Design review of the part built by this model. Coordinates are the model's own, in mm. A direction names the side the tool comes from. Round coordinates to 2 decimals unless told otherwise and drop trailing zeros. Write each loop counter-clockwise with the first axis right and the second up, starting at its lowest first coordinate (ties: lowest second). Pieces come first, ordered by that corner, then holes.
from build123d import *

# Parameters (mm, degrees)
SKETCH1_W           = 400
SKETCH1_H           = 300
BOSS_EXTRUDE1_DEPTH = 10
SKETCH2_W           = 8
SKETCH2_H           = 30
BOSS_EXTRUDE2_DEPTH = 40
SKETCH3_R           = 5
CUT_EXTRUDE1_DEPTH  = 374.607079697
FILLET1_R           = 15
SKETCH4_W           = 8
SKETCH4_H           = 30
BOSS_EXTRUDE3_DEPTH = 40
SKETCH5_R           = 5
CUT_EXTRUDE2_DEPTH  = 374.607079697
FILLET2_R           = 15


with BuildPart() as part:
    # Sketch1 → Boss-Extrude1 (new body)
    with BuildSketch(Plane(origin=(0, 0, 0), x_dir=(1, 0, 0), z_dir=(0, 1, 0))):
        Rectangle(SKETCH1_W, SKETCH1_H)
    extrude(amount=BOSS_EXTRUDE1_DEPTH)

    # Sketch2 → Boss-Extrude2 (add)
    with BuildSketch(Plane(origin=(0, 10, 0), x_dir=(1, 0, 0), z_dir=(0, 1, 0))):
        with Locations((-134.5, -130)):
            Rectangle(SKETCH2_W, SKETCH2_H)
        with Locations((-76.5, -130)):
            Rectangle(SKETCH2_W, SKETCH2_H)
        with Locations((76.5, -130)):
            Rectangle(SKETCH2_W, SKETCH2_H)
        with Locations((134.5, -130)):
            Rectangle(SKETCH2_W, SKETCH2_H)
    extrude(amount=BOSS_EXTRUDE2_DEPTH)

    # Sketch3 → Cut-Extrude1 (cut, through all)
    with BuildSketch(Plane(origin=(138.5, 0, 0), x_dir=(0, 0, -1), z_dir=(1, 0, 0))):
        with Locations((-130, 35)):
            Circle(SKETCH3_R)
    extrude(amount=-CUT_EXTRUDE1_DEPTH, mode=Mode.SUBTRACT)

    # Fillet1
    fillet1_edges = [part.edges().sort_by_distance(p)[0] for p in [
        (134.5, 50, 115),
        (134.5, 50, 145),
        (76.5, 50, 145),
        (76.5, 50, 115),
        (-76.5, 50, 115),
        (-134.5, 50, 115),
        (-76.5, 50, 145),
        (-134.5, 50, 145),
    ]]
    fillet(fillet1_edges, radius=FILLET1_R - 0.0001)  # a hair under: the kernel refuses the full size

    # Sketch4 → Boss-Extrude3 (add)
    with BuildSketch(Plane(origin=(0, 10, 0), x_dir=(1, 0, 0), z_dir=(0, 1, 0))):
        with Locations((-134.5, 20)):
            Rectangle(SKETCH4_W, SKETCH4_H)
        with Locations((-76.5, 20)):
            Rectangle(SKETCH4_W, SKETCH4_H)
        with Locations((134.5, 20)):
            Rectangle(SKETCH4_W, SKETCH4_H)
        with Locations((76.5, 20)):
            Rectangle(SKETCH4_W, SKETCH4_H)
    extrude(amount=BOSS_EXTRUDE3_DEPTH)

    # Sketch5 → Cut-Extrude2 (cut, through all)
    with BuildSketch(Plane(origin=(138.5, 0, 0), x_dir=(0, 0, -1), z_dir=(1, 0, 0))):
        with Locations((20, 35)):
            Circle(SKETCH5_R)
    extrude(amount=-CUT_EXTRUDE2_DEPTH, mode=Mode.SUBTRACT)

    # Fillet2
    fillet2_edges = [part.edges().sort_by_distance(p)[0] for p in [
        (-134.5, 50, -35),
        (-76.5, 50, -35),
        (134.5, 50, -35),
        (76.5, 50, -35),
        (-134.5, 50, -5),
        (-76.5, 50, -5),
        (76.5, 50, -5),
        (134.5, 50, -5),
    ]]
    fillet(fillet2_edges, radius=FILLET2_R - 0.0001)  # a hair under: the kernel refuses the full size


solid = part.part
1) For line 1 along Y through (x, z) = (-135, -20); line 2 along Y through (x, z) = (-8.5, 104.5); line 3 along Z through (x, y) = (-131.5, 12), list the stretches that pass through material, from the lowest coordinate up.
2) Add section A-A on y = 24. Count the separate pieces of the cut face and the enclosed holes in it, and give its area (3 significant figures).
3) Add section B-B on x = -112.5. State the section outline as (y, z) points.
4) The part is to be moulded in two halves that separate along X. For faces 5 (the face through (80.5, 29.7, -19.8)), 6 (the face through (200, 5, 2)), 7 (the face through (134.556, 39.957, -19.349)), 8 (the face through (-130.5, 29.7, 130.2)), say which applies: pulls with the +X half, pulls with the -X half, needs draft (parallel to the pull), parting line crosses it, or undercut.
5) For faces 1 (the face through (130.5, 29.7, -19.8)), 2 (the face through (-135, 22, -5)), 3 (the face through (-134.444, 39.957, -19.349)), 4 (the face through (-77, 22, -35)), list the 3-axis set-ups (+Z, -Z, +X, -X, +Y, -Y) from which the entire face can be reached by the end or side of a thin tool; tool diameter is ignored.
6) Add section C-C on z = 5.5. State the section outline as (x, y) points, and give its area (3 significant figures).
7) For P1, Ø6.5, axis at x = -76.5, y = 19.5, coming from the -Z side; P2, Ø6, axis at y = 35, z = 130, coming from the +X side; P3, Ø4, axis at y = 40.5, z = -31.5, coming from the +X side; P4, Ø9, axis at x = -77.5, y = 27, coming from the +Z side, all flat-tipped, find the tip position at first contact; note any pin that passes through.
Computed:
1. line 1: y = 0 to 30, 40 to 50
1. line 2: y = 0 to 10
1. line 3: z = -35 to -5, 115 to 145
2. separate pieces: 8
2. enclosed holes: 0
2. area: 1,920 mm2
3. outline: (0, -150) - (10, -150) - (10, 150) - (0, 150) - close
4. face 5: undercut
4. face 6: pulls with the +X half
4. face 7: needs draft
4. face 8: undercut
5. face 1: +Z, -Z, +Y
5. face 2: +X, -X, +Y
5. face 3: +X, -X
5. face 4: -Z, +X, -X, +Y
6. outline: (-200, 0) - (200, 0) - (200, 10) - (-200, 10) - close
6. area: 4,000 mm2
7. P1: stops at z = -35
7. P2: passes through
7. P3: stops at x = 138.5
7. P4: stops at z = 145
